Autodesk Inventor part; units mm, degrees
ref_plane "YZ Plane" through (0, 0, 0) normal (1, 0, 0) x (0, 1, 0)
ref_plane "XZ Plane" through (0, 0, 0) normal (0, 1, 0) x (-1, 0, 0)
ref_plane "XY Plane" through (0, 0, 0) normal (0, 0, 1) x (1, 0, 0)
sketch "Sketch1" plane through (0, 0, 0) normal (0, 0, 1) x (1, 0, 0)
  line L0 (0, 0) -> (0, 77)
  line L1 (0, 77) -> (115, 77)
  line L2 (115, 77) -> (115, 0)
  line L3 (115, 0) -> (0, 0)
  dimension "d0" = 77
  dimension "d1" = 115
extrude "Extrusion1" add sketch "Sketch1" along normal blind 3
sketch "Sketch2" plane through (0, 0, 0) normal (0, 0, -1) x (-1, 0, 0)
  line L0 (-110, 40) -> (-5, 40)
  line L1 (-5, 40) -> (-5, 37)
  line L2 (-5, 37) -> (-110, 37)
  line L3 (-110, 37) -> (-110, 40)
  line L4 (0, 77) -> (0, 0)
  line L5 (-115, 0) -> (-115, 77)
  point P0 (-5, 38.5)
  point P1 (0, 38.5)
  dimension "d4" = 3
  dimension "d5" = 5
  dimension "d6" = 5
extrude "Extrusion2" cut sketch "Sketch2" against normal blind 10
properties part number "rampa"
CAD build for the part. Positions are in the model's coordinates, mm. A direction names the side the tool comes from. Round coordinates to 2 decimals unless told otherwise and drop trailing zeros. Order: outer loops, then holes, each group sorted by start corner. A loop starts at its lowest first (then second) coordinate and runs counter-clockwise, first axis right, second up. Notation, with made-up numbers: (79.5, 65) -> (87.5, 65) arc R18 cw to (87.5, 100) -> close; hole circle Ø8 at (-1, 33). An arc over 180 degrees is marked (long way). Write item = value, one per line. Start each with the question number.
(1) Pull direction Y, two halves, no side cores. Call faces 3 (the flat face through (57, 48, 0)), 4 (the flat face through (58, 40, 1)), 5 (the flat face through (58, 0, 1)): released by +Y, released by -Y, zero draft, split by the parting line, or undercut.
(2) Pin check, flat tip, straight feed: P1, Ø1, axis at x = 97.5, y = 69, coming from the -Z side. Stop position of the tip, or through.
(3) Cut at A-A, the plane x = 77. List the corners of the cut face in (y, z).
(4) Which spindle directions (+Z, -Z, +X, -X, +Y, -Y) get a long thin tool onto all of the face, cutting with end or side? Do faces 1 (the flat face through (115, 39, 1)), 2 (the flat face through (5, 39, 1)). Say none if no direction does.
(5) Cut at B-B, the plane z = 1.2. List the corners of the cut face in (x, y).
(6) Probe line 1 (Y direction, x = 36, z = 0.1). List the from-to ranges inside material, lowest first. Write a range as [from, to].
Model answer:
q1.face_3 = zero draft
q1.face_4 = undercut
q1.face_5 = released by -Y
q2.P1 = 0
q3.outline = (0, 0) -> (37, 0) -> (37, 3) -> (0, 3) -> close; (40, 0) -> (77, 0) -> (77, 3) -> (40, 3) -> close
q4.face_1 = +Z, -Z, +X, +Y, -Y
q4.face_2 = +Z, -Z
q5.outline = (0, 0) -> (115, 0) -> (115, 77) -> (0, 77) -> close; hole (5, 37) -> (110, 37) -> (110, 40) -> (5, 40) -> close
q6.line_1 = [0, 37], [40, 77]
